Check sheet for the drawn part. Datum: minimum x, y, z corner. Units: mm. A direction names the side the tool comes from. Give positions to 0.01 mm unless a question says otherwise; leave off trailing zeros. Loops run counter-clockwise (first coordinate to the right, second up) from the corner with the lowest first, then second, coordinate; pieces in that order, holes last. Notation, with made-up numbers: (24.5, -24.75) - (52.5, -24.75) arc R24 cw to (52.5, -2.75) - close; hole circle Ø9 at (7.5, 16). An arc over 180 degrees is marked (long way). Use a Markdown table: item, result. Add a question column.
1. Material ranges on L1, parallel to X at y = 4.65, z = 12.5; L2, parallel to X at y = 1.85, z = 12.5, recorded low to high.
2. Depth check by flat-ended pin: P1, Ø3, axis at x = 21, z = 21, coming from the +Y side; P2, Ø9, axis at x = 12.5, z = 12.5, coming from the +Y side; P3, Ø4, axis at y = 4, z = 6.5, coming from the -X side. Enter the tip coordinate at first touch or a pass-through.
3. Cross-section at D-D on y = 2. Enter the section's corners in (x, z).
4. Cross-section at A-A on x = 12.5. Enter the section's corners in (y, z), and give its area (3 significant figures).
5. Cross-section at B-B on z = 12.5. Enter the section's corners in (x, y).
6. Cross-section at C-C on y = 7. Enter the section's corners in (x, z), and give its area (3 significant figures).
7. Draft check along Z on the marked faces 3, 4, 5 and 6. Enter one of: pulls with the +Z half, pulls with the -Z half, needs draft (parallel to the pull), parting line crosses it, or undercut.
8. Set-up check for the marked faces 1 and 2: record each of +Z, -Z, +X, -X, +Y, -Y from which the full face is reachable in a straight line by a thin tool's end or side.
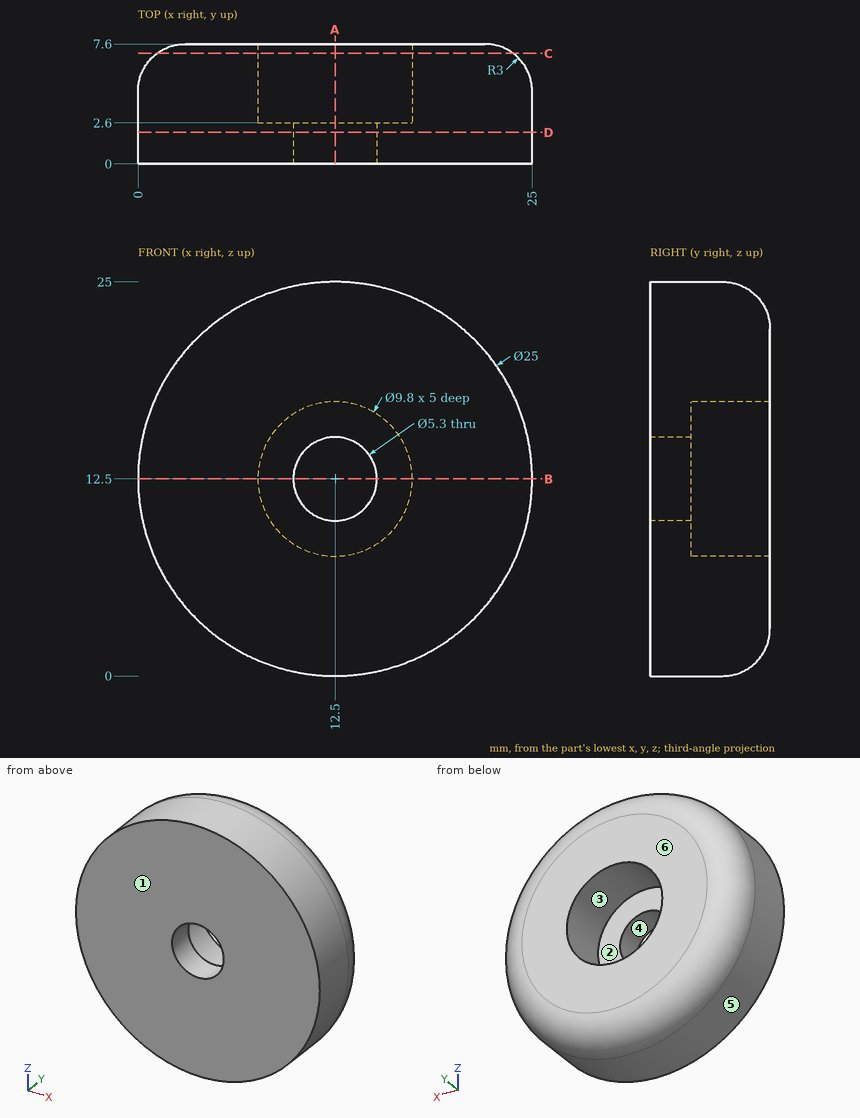
Values found:
| question | item | result |
|---|---|---|
| 1 | L1 | x = 0 to 7.6, 17.4 to 25 |
| 1 | L2 | x = 0 to 9.85, 15.15 to 25 |
| 2 | P1 | stops at y = 7.42 |
| 2 | P2 | stops at y = 2.6 |
| 2 | P3 | stops at x = 0.66 |
| 3 | outline | circle Ø25 at (12.5, 12.5); hole circle Ø5.3 at (12.5, 12.5) |
| 4 | outline | (0, 0) - (4.6, 0) arc R3 ccw to (7.6, 3) - (7.6, 7.6) - (2.6, 7.6) - (2.6, 9.85) - (0, 9.85) - close; (0, 15.15) - (2.6, 15.15) - (2.6, 17.4) - (7.6, 17.4) - (7.6, 22) arc R3 ccw to (4.6, 25) - (0, 25) - close |
| 4 | area | 123 mm2 |
| 5 | outline | (0, 0) - (9.85, 0) - (9.85, 2.6) - (7.6, 2.6) - (7.6, 7.6) - (3, 7.6) arc R3 ccw to (0, 4.6) - close; (15.15, 0) - (25, 0) - (25, 4.6) arc R3 ccw to (22, 7.6) - (17.4, 7.6) - (17.4, 2.6) - (15.15, 2.6) - close |
| 6 | outline | circle Ø22.6 at (12.5, 12.5); hole circle Ø9.8 at (12.5, 12.5) |
| 6 | area | 326 mm2 |
| 7 | face 3 | undercut |
| 7 | face 4 | undercut |
| 7 | face 5 | parting line crosses it |
| 7 | face 6 | needs draft |
| 8 | face 1 | +Z, -Z, +X, -X, -Y |
| 8 | face 2 | +Y |
